```python
from build123d import *

# Parameters (mm, degrees)
SKETCH1_R           = 2.5
SKETCH1_W           = 15
SKETCH1_H           = 2.5
BOSS_EXTRUDE1_DEPTH = 2.5
FILLET1_R           = 2


with BuildPart() as part:
    # Sketch1 → Boss-Extrude1 (new body)
    with BuildSketch(Plane(origin=(0, 0, 0), x_dir=(1, 0, 0), z_dir=(0, 1, 0))):
        with BuildLine():
            Line((35, 45), (32.5, 45))
            Line((32.5, 45), (32.5, 10))
            Line((32.5, 10), (35, 10))
            Line((35, 10), (35, -10))
            Line((35, -10), (32.5, -10))
            Line((32.5, -10), (32.5, -45))
            Line((32.5, -45), (35, -45))
            Line((35, -45), (35, -65))
            Line((35, -65), (32.5, -65))
            Line((32.5, -65), (32.5, -75))
            Line((32.5, -75), (15, -75))
            ThreePointArc((15, -75), (0, -90), (-15, -75))
            Line((-15, -75), (-32.5, -75))
            Line((-32.5, -75), (-32.5, -65))
            Line((-32.5, -65), (-35, -65))
            Line((-35, -65), (-35, -45))
            Line((-35, -45), (-32.5, -45))
            Line((-32.5, -45), (-32.5, -10))
            Line((-32.5, -10), (-35, -10))
            Line((-35, -10), (-35, 10))
            Line((-35, 10), (-32.5, 10))
            Line((-32.5, 10), (-32.5, 45))
            Line((-32.5, 45), (-35, 45))
            Line((-35, 45), (-35, 65))
            Line((-35, 65), (-32.5, 65))
            Line((-32.5, 65), (-32.5, 70.5))
            Line((-32.5, 70.5), (-25, 70.5))
            Line((-25, 70.5), (-25, 73))
            Line((-25, 73), (-10, 73))
            Line((-10, 73), (-10, 70.5))
            Line((-10, 70.5), (10, 70.5))
            Line((10, 70.5), (10, 73))
            Line((10, 73), (25, 73))
            Line((25, 73), (25, 70.5))
            Line((25, 70.5), (32.5, 70.5))
            Line((32.5, 70.5), (32.5, 65))
            Line((32.5, 65), (35, 65))
            Line((35, 65), (35, 45))
        make_face()
        with Locations(Location((0, -80, 0), (0, 0, 270))):
            Circle(SKETCH1_R, mode=Mode.SUBTRACT)
        with Locations((17.5, 0)):
            Rectangle(SKETCH1_W, SKETCH1_H, mode=Mode.SUBTRACT)
        with Locations((-17.5, 0)):
            Rectangle(SKETCH1_W, SKETCH1_H, mode=Mode.SUBTRACT)
        with Locations((-17.5, -71.75)):
            Rectangle(SKETCH1_W, SKETCH1_H, mode=Mode.SUBTRACT)
        with Locations((17.5, -71.75)):
            Rectangle(SKETCH1_W, SKETCH1_H, mode=Mode.SUBTRACT)
    extrude(amount=BOSS_EXTRUDE1_DEPTH)

    # Fillet1
    fillet1_edges = [part.edges().sort_by_distance(p)[0] for p in [
        (15, 1.25, 75),
        (-15, 1.25, 75),
    ]]
    fillet(fillet1_edges, radius=FILLET1_R)


solid = part.part
```
The model under review builds one solid part; all positions refer to its coordinate system, in mm. Give positions to 0.01 mm unless a question says otherwise; leave off trailing zeros. Order: outer loops, then holes, each group sorted by start corner. A loop starts at its lowest first (then second) coordinate and runs counter-clockwise, first axis right, second up. Notation, with made-up numbers: (-3.75, -8.5) - (36.25, -8.5) arc R15 cw to (36.25, 18.5) - close; hole circle Ø6 at (67, 23). An arc over 180 degrees is marked (long way). Use CSV: the item, a comma, the result in double quotes. Start each with the question number.
Q1. Clearance check with flat-ended pins moving along their axes: pin 1 Ø0.8 at (x, y) = (-34, 1.5) entering from +Z; pin 2 Ø1.2 at (y, z) = (1, -25) entering from +X; pin 3 Ø0.8 at (x, y) = (27.5, 1.5) entering from -Z. State where each tip first meets the part, or that it passes through.
Q2. We need section B-B, the plane x = 0. Write out the cut boundary in (y, z).
Q3. We need section A-A, the plane x = -23.5. Write out the cut boundary in (y, z), and give its area (4 significant figures).
Q4. The part is to be moulded in two halves that separate along Z. For faces 1 (the cylindrical face through (0, 1, 90)), 2 (the flat face through (0, 2.5, 7)), 3 (the cylindrical face through (0.1, 1.2, 77.5)), say which applies: +Z half, -Z half, draft (parallel to the pull), parting line (faces both ways), or undercut.
Q5. To check wall thickness, follow line 1 along Z through (x, y) = (24.5, 1.75); line 2 along X through (y, z) = (2.3, 26.5); line 3 along Z through (x, y) = (28, 1.5). State the ranges of each line that lie inside material, in increasing order. Write a range as [from, to].
Q6. We need section C-C, the plane z = 80. Write out the cut boundary in (x, y), and give its area (3 significant figures).
Q7. We need section D-D, the plane y = 0.6. State how many separate pieces and enclosed holes the cut face has, and give its area (3 significant figures).
Outcome:
1,pin 1,"stops at z = 65"
1,pin 2,"stops at x = 32.5"
1,pin 3,"stops at z = -70.5"
2,outline,"(0, -70.5) - (2.5, -70.5) - (2.5, 77.5) - (0, 77.5) - close; (0, 82.5) - (2.5, 82.5) - (2.5, 90) - (0, 90) - close"
3,outline,"(0, -73) - (2.5, -73) - (2.5, -1.25) - (0, -1.25) - close; (0, 1.25) - (2.5, 1.25) - (2.5, 70.5) - (0, 70.5) - close; (0, 73) - (2.5, 73) - (2.5, 75) - (0, 75) - close"
3,area,"357.5 mm^2"
4,face 1,"+Z half"
4,face 2,"draft"
4,face 3,"undercut"
5,line 1,"z = [-73, -1.25], [1.25, 70.5], [73, 75]"
5,line 2,"x = [-32.5, 32.5]"
5,line 3,"z = [-70.5, 75]"
6,outline,"(-14.14, 0) - (-2.5, 0) - (-2.5, 2.5) - (-14.14, 2.5) - close; (2.5, 0) - (14.14, 0) - (14.14, 2.5) - (2.5, 2.5) - close"
6,area,"58.2 mm^2"
7,separate pieces,"1"
7,enclosed holes,"5"
7,area,"10,000 mm^2"
